Design review of the part built by this model. Coordinates are the model's own, in mm. A direction names the side the tool comes from. Round coordinates to 2 decimals unless told otherwise and drop trailing zeros. Loops run counter-clockwise (first coordinate to the right, second up) from the corner with the lowest first, then second, coordinate; pieces in that order, holes last. Notation, with made-up numbers: (9.5, 6.25) -> (61.5, 6.25) arc R16 cw to (61.5, 14.25) -> close; hole circle Ø11 at (12, -22). An arc over 180 degrees is marked (long way). Use a Markdown table: item, result. Add a question column.
from build123d import *

# Parameters (mm, degrees)
SKETCH2_W               = 64.4
SKETCH2_H               = 24.4
BOSS_EXTRUDE1_DEPTH     = 20
SKETCH3_W               = 58
SKETCH3_H               = 18
CUT_EXTRUDE1_DEPTH      = 18
FILLET1_R               = 1
SKETCH4_W               = 1
SKETCH4_H               = 3.96
CUT_EXTRUDE2_DEPTH      = 4
SKETCH5_W               = 1.6
SKETCH5_H               = 3.96
CUT_EXTRUDE3_DEPTH      = 12
MIRROR5_COPY_1_SKETCH_W = 1
MIRROR5_COPY_1_SKETCH_H = 3.96
MIRROR5_COPY_1_DEPTH    = 4
MIRROR5_COPY_2_SKETCH_W = 1.6
MIRROR5_COPY_2_SKETCH_H = 3.96
MIRROR5_COPY_2_DEPTH    = 12
CUT_EXTRUDE4_REACH      = 70.529
SKETCH6_R               = 0.75


with BuildPart() as part:
    # Sketch2 → Boss-Extrude1 (new body)
    with BuildSketch(Plane(origin=(0, 0, 0), x_dir=(1, 0, 0), z_dir=(0, 1, 0))):
        Rectangle(SKETCH2_W, SKETCH2_H)
    extrude(amount=BOSS_EXTRUDE1_DEPTH)

    # Sketch3 → Cut-Extrude1 (cut)
    with BuildSketch(Plane(origin=(0, 20, 0), x_dir=(1, 0, 0), z_dir=(0, 1, 0))):
        Rectangle(SKETCH3_W, SKETCH3_H)
    extrude(amount=-CUT_EXTRUDE1_DEPTH, mode=Mode.SUBTRACT)

    # Fillet1
    fillet1_edges = [part.edges().sort_by_distance(p)[0] for p in [
        (32.2, 10, 12.2),
        (-32.2, 10, 12.2),
        (-32.2, 10, -12.2),
        (32.2, 10, -12.2),
    ]]
    fillet(fillet1_edges, radius=FILLET1_R)

    # Sketch4 → Cut-Extrude2 (cut)
    with BuildSketch(Plane(origin=(0, 20, 0), x_dir=(1, 0, 0), z_dir=(0, 1, 0))):
        with Locations((-29.5, 1.98)):
            Rectangle(SKETCH4_W, SKETCH4_H)
    cut_extrude2 = extrude(amount=-CUT_EXTRUDE2_DEPTH, mode=Mode.SUBTRACT)

    # Sketch5 → Cut-Extrude3 (cut)
    with BuildSketch(Plane(origin=(0, 20, 0), x_dir=(1, 0, 0), z_dir=(0, 1, 0))):
        with Locations((-30.8, 1.98)):
            Rectangle(SKETCH5_W, SKETCH5_H)
    cut_extrude3 = extrude(amount=-CUT_EXTRUDE3_DEPTH, mode=Mode.SUBTRACT)

    # Mirror4: Cut-Extrude2, Cut-Extrude3 across plane
    add(cut_extrude2.mirror(Plane(origin=(0, 0, 0), x_dir=(0, 0, 1), z_dir=(1, 0, 0))), mode=Mode.SUBTRACT)
    add(cut_extrude3.mirror(Plane(origin=(0, 0, 0), x_dir=(0, 0, 1), z_dir=(1, 0, 0))), mode=Mode.SUBTRACT)

    # Mirror5: Cut-Extrude2, Cut-Extrude3 across plane
    add(cut_extrude2.mirror(Plane.XY), mode=Mode.SUBTRACT)
    add(cut_extrude3.mirror(Plane.XY), mode=Mode.SUBTRACT)

    # Mirror5 copy 1 sketch → Mirror5 copy 1 (cut)
    with BuildSketch(Plane(origin=(0, 20, 0), x_dir=(-1, 0, 0), z_dir=(0, 1, 0))):
        with Locations((-29.5, 1.98)):
            Rectangle(MIRROR5_COPY_1_SKETCH_W, MIRROR5_COPY_1_SKETCH_H)
    extrude(amount=-MIRROR5_COPY_1_DEPTH, mode=Mode.SUBTRACT)

    # Mirror5 copy 2 sketch → Mirror5 copy 2 (cut)
    with BuildSketch(Plane(origin=(0, 20, 0), x_dir=(-1, 0, 0), z_dir=(0, 1, 0))):
        with Locations((-30.8, 1.98)):
            Rectangle(MIRROR5_COPY_2_SKETCH_W, MIRROR5_COPY_2_SKETCH_H)
    extrude(amount=-MIRROR5_COPY_2_DEPTH, mode=Mode.SUBTRACT)

    # Sketch6 → Cut-Extrude4 (cut, up to next)
    with BuildSketch(Plane(origin=(32.2, 0, 0), x_dir=(0, 0, -1), z_dir=(1, 0, 0)), mode=Mode.PRIVATE) as cut_extrude4_sk1:
        with Locations((0, 10)):
            Circle(SKETCH6_R)
    cut_extrude4_tool1 = extrude(cut_extrude4_sk1.sketch, amount=-CUT_EXTRUDE4_REACH, mode=Mode.PRIVATE) & part.part
    cut_extrude4 = cut_extrude4_tool1.solids().sort_by_distance((32.2, 10, 0))[0]
    add(cut_extrude4, mode=Mode.SUBTRACT)

    # Mirror6: Cut-Extrude4 across plane
    add(cut_extrude4.mirror(Plane(origin=(0, 0, 0), x_dir=(0, 0, 1), z_dir=(1, 0, 0))), mode=Mode.SUBTRACT)


solid = part.part
1. For faces 1 (the face through (-31.904, 10.744, 0.098)), 2 (the face through (31, 8, 0)), 3 (the face through (0, 10, -12.2)), list the 3-axis set-ups (+Z, -Z, +X, -X, +Y, -Y) from which the entire face can be reached by the end or side of a thin tool; tool diameter is ignored.
2. Mouldability with a two-part tool opening along X and no side actions: class faces 4 (the face through (30, 12, 0)), 5 (the face through (0, 0, 0)), 6 (the face through (32.2, 12, 0)) as +X half, -X half, draft (parallel to the pull), parting line (faces both ways), or undercut.
3. To check wall thickness, follow probe 1 along X at (y, z) = (8.75, 0.5); probe 2 along X at (y, z) = (2.75, -2.25); probe 3 along Z at (x, y) = (14, 9.5). State the ranges of each line that lie inside material, in increasing order. Write a range as from..to.
4. Consider section D-D on z = 7.5. State the section outline as (x, y) points, plus the area to 3 significant figures.
5. Consider section A-A on z = 0. State the section outline as (x, y) points, plus the area to 3 significant figures.
6. Consider section C-C on y = 11.75. State the section outline as (x, z) points, plus the area to 3 significant figures.
7. Consider section B-B on y = 6.5. State the section outline as (x, z) points, plus the area to 3 significant figures.
8. Insertion check: P1, Ø12, axis at x = -21.5, z = 2.5, coming from the +Y side; P2, Ø0.5, axis at x = 29.5, z = 1, coming from the +Y side; P3, Ø0.5, axis at x = 31, z = -1, coming from the +Y side. Each pin has a flat end and moves straight along its axis. Give the tip position at first contact, or say it passes through.
Verdict:
| question | item | result |
|---|---|---|
| 1 | face 1 | -X |
| 1 | face 2 | +Y |
| 1 | face 3 | -Z, +X, -X, +Y, -Y |
| 2 | face 4 | undercut |
| 2 | face 5 | draft |
| 2 | face 6 | +X half |
| 3 | probe 1 | x = -32.2..-31.6, -30..-29, 29..30, 31.6..32.2 |
| 3 | probe 2 | x = -32.2..-29, 29..32.2 |
| 3 | probe 3 | z = -12.2..-9, 9..12.2 |
| 4 | outline | (-32.2, 0) -> (32.2, 0) -> (32.2, 20) -> (29, 20) -> (29, 2) -> (-29, 2) -> (-29, 20) -> (-32.2, 20) -> close |
| 4 | area | 244 mm² |
| 5 | outline | (-32.2, 0) -> (32.2, 0) -> (32.2, 9.25) -> (31.6, 9.25) -> (31.6, 8) -> (30, 8) -> (30, 16) -> (29, 16) -> (29, 2) -> (-29, 2) -> (-29, 16) -> (-30, 16) -> (-30, 8) -> (-31.6, 8) -> (-31.6, 9.25) -> (-32.2, 9.25) -> close; (-32.2, 10.75) -> (-31.6, 10.75) -> (-31.6, 20) -> (-32.2, 20) -> close; (31.6, 10.75) -> (32.2, 10.75) -> (32.2, 20) -> (31.6, 20) -> close |
| 5 | area | 196 mm² |
| 6 | outline | (-32.2, -11.2) arc R1 ccw to (-31.2, -12.2) -> (31.2, -12.2) arc R1 ccw to (32.2, -11.2) -> (32.2, 11.2) arc R1 ccw to (31.2, 12.2) -> (-31.2, 12.2) arc R1 ccw to (-32.2, 11.2) -> close; hole (-31.6, -3.96) -> (-30, -3.96) -> (-30, 3.96) -> (-31.6, 3.96) -> close; hole (-29, -9) -> (29, -9) -> (29, 9) -> (-29, 9) -> close; hole (30, -3.96) -> (31.6, -3.96) -> (31.6, 3.96) -> (30, 3.96) -> close |
| 6 | area | 501 mm² |
| 7 | outline | (-32.2, -11.2) arc R1 ccw to (-31.2, -12.2) -> (31.2, -12.2) arc R1 ccw to (32.2, -11.2) -> (32.2, 11.2) arc R1 ccw to (31.2, 12.2) -> (-31.2, 12.2) arc R1 ccw to (-32.2, 11.2) -> close; hole (-29, -9) -> (29, -9) -> (29, 9) -> (-29, 9) -> close |
| 7 | area | 527 mm² |
| 8 | P1 | stops at y = 2 |
| 8 | P2 | stops at y = 16 |
| 8 | P3 | stops at y = 8 |
